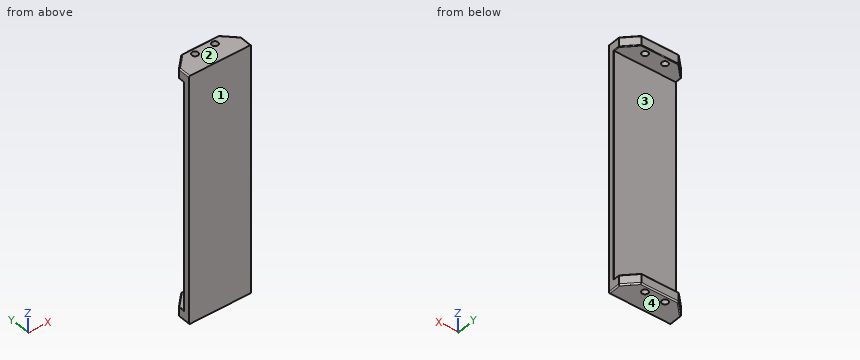
```python
from build123d import *

# Parameters (mm, degrees)
SKETCH1_W           = 500
SKETCH1_H           = 200
BOSS_EXTRUDE1_DEPTH = 2000
SKETCH3_W           = 1840
SKETCH3_H           = 150
CUT_EXTRUDE1_DEPTH  = 1000
CUT_EXTRUDE2_DEPTH  = 2001
SKETCH4_R           = 25
CUT_EXTRUDE3_DEPTH  = 2001
FILLET1_R           = 10
FILLET2_R           = 10
FILLET4_R           = 5


with BuildPart() as part:
    # Sketch1 → Boss-Extrude1 (new body)
    with BuildSketch(Plane.XY):
        Rectangle(SKETCH1_W, SKETCH1_H)
    extrude(amount=BOSS_EXTRUDE1_DEPTH)

    # Sketch3 → Cut-Extrude1 (cut)
    with BuildSketch(Plane.ZY.offset(250)):
        with Locations((1000, 25)):
            Rectangle(SKETCH3_W, SKETCH3_H)
    extrude(amount=-CUT_EXTRUDE1_DEPTH, mode=Mode.SUBTRACT)

    # Sketch2 → Cut-Extrude2 (cut, through all)
    with BuildSketch(Plane.XY.offset(2000)):
        Polygon((-250, 0), (-150, 100), (-250, 100), align=None)
        Polygon((250, 0), (150, 100), (250, 100), align=None)
    extrude(amount=-CUT_EXTRUDE2_DEPTH, mode=Mode.SUBTRACT)

    # Sketch4 → Cut-Extrude3 (cut, through all)
    with BuildSketch(Plane.XY.offset(2000)):
        with Locations((-80, 50)):
            Circle(SKETCH4_R)
        with Locations((80, 50)):
            Circle(SKETCH4_R)
    extrude(amount=-CUT_EXTRUDE3_DEPTH, mode=Mode.SUBTRACT)

    # Fillet1
    fillet1_edges = [part.edges().sort_by_distance(p)[0] for p in [
        (-250, -50, 2000),
        (250, -50, 2000),
        (-200, 50, 2000),
        (0, 100, 2000),
        (200, 50, 2000),
    ]]
    fillet(fillet1_edges, radius=FILLET1_R)

    # Fillet2
    fillet2_edges = [part.edges().sort_by_distance(p)[0] for p in [
        (-250, -50, 0),
        (-200, 50, 0),
        (0, 100, 0),
        (250, -50, 0),
        (200, 50, 0),
    ]]
    fillet(fillet2_edges, radius=FILLET2_R)

    # Fillet4
    fillet4_edges = [part.edges().sort_by_distance(p)[0] for p in [
        (250, -25, 1920),
        (250, -50, 1000),
        (-250, -50, 1000),
        (-250, -25, 1920),
        (-200, 50, 1920),
        (-250, -25, 80),
        (-200, 50, 80),
        (0, 100, 1920),
        (200, 50, 1920),
        (0, 100, 80),
        (250, -25, 80),
        (200, 50, 80),
    ]]
    fillet(fillet4_edges, radius=FILLET4_R)


solid = part.part
```
Source: CAD feature listing. Evaluate the final solid. Frame: model axes, mm. Face numbers are marked on the shaded views. Coordinates: 2 decimals unless noted, no trailing zeros. Order: outer loops, then holes, each group sorted by start corner. A loop starts at its lowest first (then second) coordinate and runs counter-clockwise, first axis right, second up. Notation, with made-up numbers: M 53.5,-26 L 83.5,-26 A12 cw 83.5,-18 Z; hole C 74,89 d3. An arc over 180 degrees is marked long. Write each question's results on one line, items separated by ' | '. Start each with the question number.
1) Section query D-D (y = 50). Give the number of separate pieces and of enclosed holes in the cut face, plus the area to 3 significant figures.
2) Draft query along Z for the marked faces 1, 2, 3 and 4. Return one class per face: released by +Z, released by -Z, zero draft, split by the parting line, or undercut.
3) Section query A-A (x = -80). Return the cut outline in (y, z).
4) Line query: line 1 (Y direction, x = -80, z = 1941); line 2 (Z direction, x = -3.5, y = -17); line 3 (Y direction, x = -30, z = 403.5). Output: solid intervals per line, ascending. Write a range as from..to.
5) Section query B-B (x = 24.5). Return the cut outline in (y, z), plus the area to 3 significant figures.
6) Contact query for a flat-ended pin moving along its axis: pin 1 Ø10 at (x, z) = (115, 484) entering from +Y. Output: stop coordinate, or through.
7) Section query C-C (z = 816.5). Return the cut outline in (x, y), plus the area to 3 significant figures.
Answers:
1) separate pieces: 6 | enclosed holes: 0 | area: 47,800 mm^2
2) face 1: zero draft | face 2: released by +Z | face 3: undercut | face 4: released by -Z
3) outline: M -100,0 L 25,0 L 25,80 L -50,80 L -50,1920 L 25,1920 L 25,2000 L -100,2000 Z; M 75,0 L 90,0 A10 ccw 100,10 L 100,75 A5 ccw 95,80 L 75,80 Z; M 75,1920 L 95,1920 A5 ccw 100,1925 L 100,1990 A10 ccw 90,2000 L 75,2000 Z
4) line 1: y = -100..25, 75..100 | line 2: z = 0..80, 1920..2000 | line 3: y = -100..-50
5) outline: M -100,0 L 90,0 A10 ccw 100,10 L 100,75 A5 ccw 95,80 L -50,80 L -50,1920 L 95,1920 A5 ccw 100,1925 L 100,1990 A10 ccw 90,2000 L -100,2000 Z | area: 124,000 mm^2
6) pin 1: stops at y = -50
7) outline: M -250,-100 L 250,-100 L 250,-55 A5 ccw 245,-50 L -245,-50 A5 ccw -250,-55 Z | area: 25,000 mm^2
